from build123d import *

# Parameters (mm, degrees)
F0_R     = 17.5
F1_DEPTH = 4
F2_R     = 17.5
F2_R_2   = 15.5
F3_DEPTH = 1
F4_R     = 15.5
F5_DEPTH = 25


with BuildPart() as f1:
    # F0 (on Top) → F1 (new body)
    with BuildSketch(Plane.XY):
        Circle(F0_R)
    extrude(amount=F1_DEPTH)

    # F2 (on face) → F3 (join)
    with BuildSketch(Plane.XY.offset(4)):
        Circle(F2_R)
        Circle(F2_R_2, mode=Mode.SUBTRACT)
    extrude(amount=F3_DEPTH)

    # F4 (on face) → F5 (intersect)
    with BuildSketch(Plane.XY.offset(5)):
        with BuildLine():
            ThreePointArc((2.0529786403, 17.3791621979), (0, 16.8999925429), (-2.0529786403, 17.3791621979))
            ThreePointArc((-2.0529786403, 17.3791621979), (-11.6258951009, -13.0800826872), (17.5, 0))
            ThreePointArc((17.5, 0), (13.0800826872, 11.6258951009), (2.0529786403, 17.3791621979))
        make_face()
        Circle(F4_R, mode=Mode.SUBTRACT)
        Circle(F4_R)
    extrude(amount=-F5_DEPTH, mode=Mode.INTERSECT)


solid = f1.part
Could you check a few things on this model? Use its own coordinates, in mm. A direction names the side the tool comes from. Give positions to 0.01 mm unless a question says otherwise; leave off trailing zeros. Order: outer loops, then holes, each group sorted by start corner. A loop starts at its lowest first (then second) coordinate and runs counter-clockwise, first axis right, second up.
Item 1: If we section it at B-B, the plane y = 0: Write out the boundary of the cut face in (x, z), plus the area to 3 significant figures.
Item 2: If we section it at A-A, the plane x = 0: Write out the boundary of the cut face in (y, z).
Item 3: I'm going to push flat-ended pins straight in: pin 1 (4 mm diameter, centred on x = 13, y = 2.5, fed in from +Z); pin 2 (3 mm diameter, centred on x = 5.5, z = 3.5, fed in from +Y); pin 3 (1 mm diameter, centred on y = -5, z = 4, fed in from +X). Where does each tip first touch, or does it pass through?
Item 4: I need wall thicknesses on line 1 (Y direction, x = 0, z = 4.4); line 2 (Z direction, x = -15, y = -3); line 3 (X direction, y = 11, z = 4.25). Which ranges of each line are inside material? Lowest first, please.
Item 5: For faces 4 (the face through (0, 0, 0)), 5 (the face through (0, 0, 4)), which set-ups out of +Z, -Z, +X, -X, +Y, -Y let a thin tool reach every point of the face, with its end or its side?
Item 6: If we section it at C-C, the plane z = 2.95: Write out the boundary of the cut face in (x, y), plus the area to 3 significant figures.
Item 7: If we mould it in two halves opening along X, with no side actions, what happens to faces 1 (the face through (-2.018, 15.368, 4.493)), 2 (the face through (-0.741, -17.484, 2.465)), 3 (the face through (0, 16, 5))? For each: pulls with the +X half, pulls with the -X half, needs draft (parallel to the pull), parting line crosses it, or undercut.
Values:
1. outline: (-17.5, 0) - (17.5, 0) - (17.5, 5) - (15.5, 5) - (15.5, 4) - (-15.5, 4) - (-15.5, 5) - (-17.5, 5) - close
1. area: 144 mm2
2. outline: (-17.5, 0) - (16.9, 0) - (16.9, 5) - (15.5, 5) - (15.5, 4) - (-15.5, 4) - (-15.5, 5) - (-17.5, 5) - close
3. pin 1: stops at z = 4
3. pin 2: stops at y = 17.04
3. pin 3: stops at x = 16.91
4. line 1: y = -17.5 to -15.5, 15.5 to 16.9
4. line 2: z = 0 to 4
4. line 3: x = -13.61 to -10.92, 10.92 to 13.61
5. face 4: -Z, +X, -X, +Y, -Y
5. face 5: +Z
6. outline: (-2.05, 17.38) arc R17.5 ccw (long way) to (2.05, 17.38) arc R4.64 cw to start
6. area: 960 mm2
7. face 1: undercut
7. face 2: parting line crosses it
7. face 3: needs draft
